Work out the finished part from the listing and answer in its coordinate system (mm). Face numbers are marked on the shaded views. Round coordinates to 2 decimals unless told otherwise and drop trailing zeros. Loops run counter-clockwise (first coordinate to the right, second up) from the corner with the lowest first, then second, coordinate; pieces in that order, holes last.
```python
from build123d import *

# Parameters (mm, degrees)
SKETCH1_R                            = 2
BOSS_EXTRUDE3_DEPTH                  = 12
SKETCH3_R                            = 4
BOSS_EXTRUDE4_DEPTH                  = 34
SKETCH4_W                            = 4
SKETCH4_H                            = 1.5
SKETCH4_W_2                          = 12
CUT_EXTRUDE1_DEPTH                   = 17
F_3_2_3_2_DIAMETER_HOLE1_D           = 3.2
F_3_2_3_2_DIAMETER_HOLE1_DEPTH       = 14
F_3_2_3_2_DIAMETER_HOLE1_CSINK_D     = 3.25
F_3_2_3_2_DIAMETER_HOLE1_CSINK_ANGLE = 90
F_3_2_3_2_DIAMETER_HOLE1_TIP         = 0.96137699
CHAMFER1_SIZE                        = 0.5


with BuildPart() as part:
    # Sketch1 → Boss-Extrude3 (new body)
    with BuildSketch(Plane.XY):
        Circle(SKETCH1_R)
    extrude(amount=-BOSS_EXTRUDE3_DEPTH)

    # Sketch3 → Boss-Extrude4 (add)
    with BuildSketch(Plane.XY):
        Circle(SKETCH3_R)
    extrude(amount=BOSS_EXTRUDE4_DEPTH)

    # Sketch4 → Cut-Extrude1 (cut, symmetric)
    with BuildSketch(Plane(origin=(0, 0, 0), x_dir=(0, 0, -1), z_dir=(1, 0, 0))):
        with Locations((-22.5, 3.25)):
            Rectangle(SKETCH4_W, SKETCH4_H)
        with Locations((-18.5, -3.25)):
            Rectangle(SKETCH4_W_2, SKETCH4_H)
    extrude(amount=CUT_EXTRUDE1_DEPTH, both=True, mode=Mode.SUBTRACT)

    # Ø3.2 (3.2) Diameter Hole1
    with Locations(Plane.XY.offset(34)):
        with Locations((0, 0)):
            CounterSinkHole(F_3_2_3_2_DIAMETER_HOLE1_D / 2, F_3_2_3_2_DIAMETER_HOLE1_CSINK_D / 2, depth=F_3_2_3_2_DIAMETER_HOLE1_DEPTH, counter_sink_angle=F_3_2_3_2_DIAMETER_HOLE1_CSINK_ANGLE)
            with Locations((0, 0, -(F_3_2_3_2_DIAMETER_HOLE1_DEPTH + F_3_2_3_2_DIAMETER_HOLE1_TIP / 2))):  # 118° drill point
                Cone(0, F_3_2_3_2_DIAMETER_HOLE1_D / 2, F_3_2_3_2_DIAMETER_HOLE1_TIP, mode=Mode.SUBTRACT)

    # Chamfer1
    chamfer1_edges = [part.edges().sort_by_distance(p)[0] for p in [
        (-2, 0, -12),
    ]]
    chamfer(chamfer1_edges, length=CHAMFER1_SIZE)


solid = part.part
```
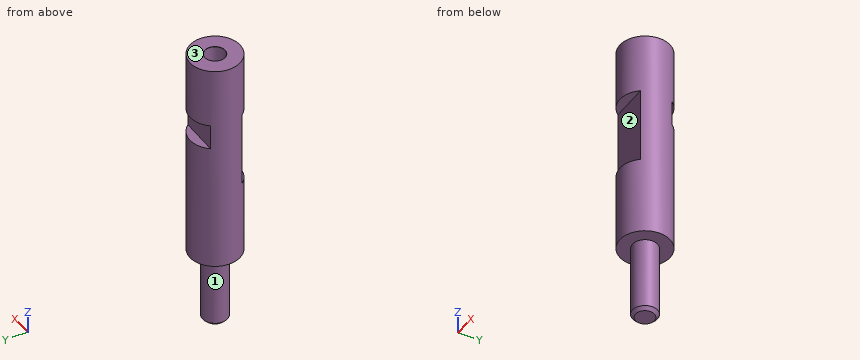
1. Find section B-B (z = 2.5). Write down the section's boundary in (x, y), then the cut area to 3 significant figures.
Answer key:
outline: circle Ø8 at (0, 0)
area: 50.3 mm2
2. Find section D-D (z = 17). Write down the section's boundary in (x, y).
Answer key:
outline: (-3.12, -2.5) - (3.12, -2.5) arc R4 ccw (long way) to start
3. Given pin 1 (1.2 mm diameter, centred on x = 0, z = 22.5, fed in from +Y); pin 2 (1.6 mm diameter, centred on x = -0.5, y = -3, fed in from -Z); pin 3 (3 mm diameter, centred on x = 1, z = 18, fed in from -Y), each flat-ended and moving along its own axis, determine where each tip first touches the part or whether it passes through.
Answer key:
pin 1: stops at y = 2.5
pin 2: stops at z = 0
pin 3: stops at y = -2.5
4. Find section A-A (z = 23.5). Write down the section's boundary in (x, y).
Answer key:
outline: (-3.12, -2.5) - (3.12, -2.5) arc R4 ccw to (3.12, 2.5) - (-3.12, 2.5) arc R4 ccw to start; hole circle Ø3.2 at (0, 0)
5. Determine the mould class of the marked faces 1, 2 and 3 for opening direction Z: +Z half, -Z half, draft (parallel to the pull), parting line (faces both ways), or undercut.
Answer key:
face 1: draft
face 2: undercut
face 3: +Z half
6. Find section C-C (z = 30). Write down the section's boundary in (x, y), then the cut area to 3 significant figures.
Answer key:
outline: circle Ø8 at (0, 0); hole circle Ø3.2 at (0, 0)
area: 42.2 mm2
7. Consider probe 1 along Z at (x, y) = (2.75, 2.75); probe 2 along Z at (x, y) = (-1.75, -3.5); probe 3 along Y at (x, z) = (0, 28.5). Determine where each line is inside the solid, lowest interval first.
Answer key:
probe 1: z = 0 to 20.5, 24.5 to 34
probe 2: z = 0 to 12.5, 24.5 to 34
probe 3: y = -4 to -1.6, 1.6 to 4
